from build123d import *

# Parameters (mm, degrees)
ESBO_O2_R                      = 27.5
RESSALTO_EXTRUS_O1_DEPTH       = 60
ESBO_O3_R                      = 27
CORTE_EXTRUS_O3_DEPTH          = 59
CORTE_EXTRUS_O3_DEPTH_BACK     = 2
ESBO_O4_R                      = 25
RESSALTO_EXTRUS_O10_DEPTH      = 69
CORTE_EXTRUS_O4_DEPTH          = 43
CORTE_EXTRUS_O4_DEPTH_BACK     = 48
RESSALTO_EXTRUS_O11_DEPTH      = 20
RESSALTO_EXTRUS_O11_DEPTH_BACK = 20
CORTE_EXTRUS_O5_DEPTH          = 30
CORTE_EXTRUS_O5_DEPTH_BACK     = 24
ESBO_O10_R                     = 25.877915993
CORTE_EXTRUS_O6_DEPTH          = 59
ESBO_O11_W                     = 32
ESBO_O11_H                     = 36
CORTE_EXTRUS_O7_DEPTH          = 68
CORTE_EXTRUS_O7_DEPTH_BACK     = 1
CORTE_EXTRUS_O10_DEPTH         = 15
CORTE_EXTRUS_O10_DEPTH_BACK    = 15
ESBO_O13_W                     = 7
ESBO_O13_H                     = 7
CORTE_EXTRUS_O11_DEPTH         = 83


with BuildPart() as part:
    # Esbo_o2 → Ressalto-extrus_o1 (new body)
    with BuildSketch(Plane.XY):
        Circle(ESBO_O2_R)
    extrude(amount=RESSALTO_EXTRUS_O1_DEPTH)

    # Esbo_o3 → Corte-extrus_o3 (cut, two sides)
    with BuildSketch(Plane.XY) as corte_extrus_o3_sk:
        Circle(ESBO_O3_R)
    extrude(amount=CORTE_EXTRUS_O3_DEPTH, mode=Mode.SUBTRACT)
    extrude(corte_extrus_o3_sk.sketch, amount=-CORTE_EXTRUS_O3_DEPTH_BACK, mode=Mode.SUBTRACT)

    # Esbo_o4 → Ressalto-extrus_o10 (add)
    with BuildSketch(Plane.XY):
        Circle(ESBO_O4_R)
    extrude(amount=RESSALTO_EXTRUS_O10_DEPTH)

    # Esbo_o6 → Corte-extrus_o4 (cut, two sides)
    with BuildSketch(Plane(origin=(0, 0, 0), x_dir=(1, 0, 0), z_dir=(0, 1, 0))) as corte_extrus_o4_sk:
        Polygon((-27.667910376, -60), (-19.667910376, -60), (-16.667910376, -69), (-27.667910376, -69), align=None)
        Polygon((27.5, -60), (19.5, -60), (16.515708897, -69), (27.5, -69), align=None)
    extrude(amount=CORTE_EXTRUS_O4_DEPTH, mode=Mode.SUBTRACT)
    extrude(corte_extrus_o4_sk.sketch, amount=-CORTE_EXTRUS_O4_DEPTH_BACK, mode=Mode.SUBTRACT)

    # Esbo_o7 → Ressalto-extrus_o11 (add, two sides)
    with BuildSketch(Plane(origin=(0, 0, 0), x_dir=(1, 0, 0), z_dir=(0, 1, 0))) as ressalto_extrus_o11_sk:
        Polygon((-4.043441925, -69), (3.891240446, -69), (9.923899261, -81), (-10.076100739, -81), align=None)
    extrude(amount=RESSALTO_EXTRUS_O11_DEPTH)
    extrude(ressalto_extrus_o11_sk.sketch, amount=-RESSALTO_EXTRUS_O11_DEPTH_BACK)

    # Esbo_o9 → Corte-extrus_o5 (cut, two sides)
    with BuildSketch(Plane(origin=(0, 0, 0), x_dir=(0, 0, -1), z_dir=(1, 0, 0))) as corte_extrus_o5_sk:
        Polygon((-81, -10.386236586), (-69, -4.386236586), (-69, -22.806779524), (-81, -22.806779524), align=None)
        Polygon((-69, 3.613763414), (-81, 9.613763414), (-81, 21.387044081), (-69, 21.387044081), align=None)
    extrude(amount=CORTE_EXTRUS_O5_DEPTH, mode=Mode.SUBTRACT)
    extrude(corte_extrus_o5_sk.sketch, amount=-CORTE_EXTRUS_O5_DEPTH_BACK, mode=Mode.SUBTRACT)

    # Esbo_o10 → Corte-extrus_o6 (cut)
    with BuildSketch(Plane.XY):
        Circle(ESBO_O10_R)
    extrude(amount=CORTE_EXTRUS_O6_DEPTH, mode=Mode.SUBTRACT)

    # Esbo_o11 → Corte-extrus_o7 (cut, two sides)
    with BuildSketch(Plane.XY) as corte_extrus_o7_sk:
        Rectangle(ESBO_O11_W, ESBO_O11_H)
    extrude(amount=CORTE_EXTRUS_O7_DEPTH, mode=Mode.SUBTRACT)
    extrude(corte_extrus_o7_sk.sketch, amount=-CORTE_EXTRUS_O7_DEPTH_BACK, mode=Mode.SUBTRACT)

    # Esbo_o12 → Corte-extrus_o10 (cut, two sides)
    with BuildSketch(Plane(origin=(0, 0, 0), x_dir=(1, 0, 0), z_dir=(0, 1, 0))) as corte_extrus_o10_sk:
        Polygon((-19.069725689, -58.817820976), (18.89199626, -58.817820976), (15.847296797, -68), (-15.94876003, -68), align=None)
    extrude(amount=CORTE_EXTRUS_O10_DEPTH, mode=Mode.SUBTRACT)
    extrude(corte_extrus_o10_sk.sketch, amount=-CORTE_EXTRUS_O10_DEPTH_BACK, mode=Mode.SUBTRACT)

    # Esbo_o13 → Corte-extrus_o11 (cut)
    with BuildSketch(Plane.XY):
        Rectangle(ESBO_O13_W, ESBO_O13_H)
    extrude(amount=CORTE_EXTRUS_O11_DEPTH, mode=Mode.SUBTRACT)


solid = part.part
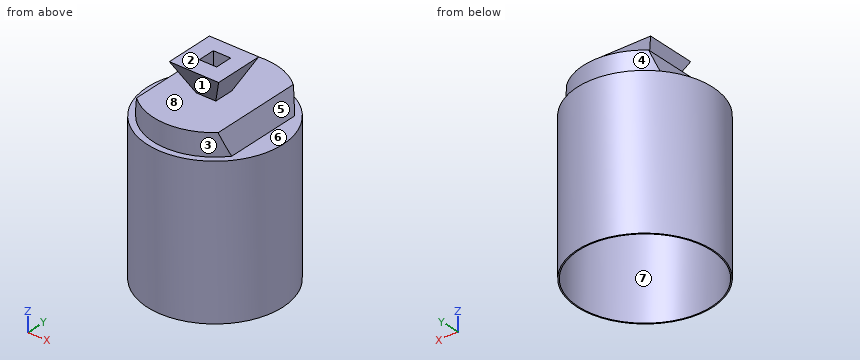
The listing builds one solid part. Answer for the finished solid, in the listing's coordinates (mm). Face numbers are marked on the shaded views. A direction names the side the tool comes from. Coordinates: 2 decimals unless noted, no trailing zeros. Write each loop counter-clockwise with the first axis right and the second up, starting at its lowest first coordinate (ties: lowest second). Pieces come first, ordered by that corner, then holes. Notation, with made-up numbers: (18, 80) -> (70, 80) arc R23 ccw to (70, 104) -> close; hole circle Ø10 at (69, 89). An arc over 180 degrees is marked (long way). One line per question, with ' | ' between items.
1. Straight lines are drawn through the part: line 1 (Y direction, x = 0, z = 20); line 2 (Y direction, x = -19, z = 40); line 3 (X direction, y = 24.5, z = 30). For each, find the intervals that lie inside material, in ascending order.
Verdict:
line 1: y = -27.5 to -27, 27 to 27.5 | line 2: y = -19.88 to -19.18, 19.18 to 19.88 | line 3: x = -12.49 to -11.35, 11.35 to 12.49
2. Section A-A (x = 0) is taken. Determine the outline of the cut face in (y, z).
Verdict:
outline: (-27.5, 0) -> (-27, 0) -> (-27, 59) -> (-18, 59) -> (-18, 68) -> (-3.5, 68) -> (-3.5, 81) -> (-10.39, 81) -> (-4.39, 69) -> (-25, 69) -> (-25, 60) -> (-27.5, 60) -> close; (3.5, 68) -> (18, 68) -> (18, 59) -> (27, 59) -> (27, 0) -> (27.5, 0) -> (27.5, 60) -> (25, 60) -> (25, 69) -> (3.61, 69) -> (9.61, 81) -> (3.5, 81) -> close
3. Section B-B (y = 0) is taken. Determine the outline of the cut face in (x, z), and give its area (3 significant figures).
Verdict:
outline: (-27.5, 0) -> (-27, 0) -> (-27, 59) -> (-19.01, 59) -> (-16, 67.85) -> (-16, 68) -> (-3.5, 68) -> (-3.5, 81) -> (-10.08, 81) -> (-4.04, 69) -> (-16.67, 69) -> (-19.67, 60) -> (-27.5, 60) -> close; (3.5, 68) -> (16, 68) -> (16, 67.54) -> (18.83, 59) -> (27, 59) -> (27, 0) -> (27.5, 0) -> (27.5, 60) -> (19.5, 60) -> (16.52, 69) -> (3.89, 69) -> (9.92, 81) -> (3.5, 81) -> close | area: 203 mm^2
4. For a pull along Z with two mould halves and no side action, classify the marked faces 6, 7 and 8 as released by +Z, released by -Z, zero draft, split by the parting line, or undercut.
Verdict:
face 6: released by +Z | face 7: zero draft | face 8: undercut
5. Section C-C (z = 14) is taken. Determine the outline of the cut face in (x, y), and give its area (3 significant figures).
Verdict:
outline: circle Ø55 at (0, 0); hole circle Ø54 at (0, 0) | area: 85.6 mm^2
6. Which of the six approach directions +Z, -Z, +X, -X, +Y, -Y give full straight-line access (tool end or side, diameter ignored) to the marked faces 1, 2, 3, 4 and 5?
Verdict:
face 1: +X, -X, -Y | face 2: +Z, +X, -X, +Y, -Y | face 3: +Z, -Y | face 4: +Z, +Y | face 5: +Z, +X, +Y, -Y
7. Section D-D (y = 13.5) is taken. Determine the outline of the cut face in (x, z).
Verdict:
outline: (-23.96, 0) -> (-23.38, 0) -> (-23.38, 59) -> (-19.01, 59) -> (-16, 67.85) -> (-16, 68) -> (16, 68) -> (16, 67.54) -> (18.83, 59) -> (23.38, 59) -> (23.38, 0) -> (23.96, 0) -> (23.96, 60) -> (19.5, 60) -> (16.52, 69) -> (-16.67, 69) -> (-19.67, 60) -> (-23.96, 60) -> close
8. Given pin 1 Ø1.5 at (x, y) = (-14.5, -13.5) entering from -Z; pin 2 Ø7.5 at (x, z) = (-0.5, 75) entering from +Y; pin 3 Ø10 at (x, z) = (5.5, 63) entering from -Y, each flat-ended and moving along its own axis, determine where each tip first touches the part or whether it passes through.
Verdict:
pin 1: stops at z = 68 | pin 2: stops at y = 8.49 | pin 3: stops at y = -27.46
